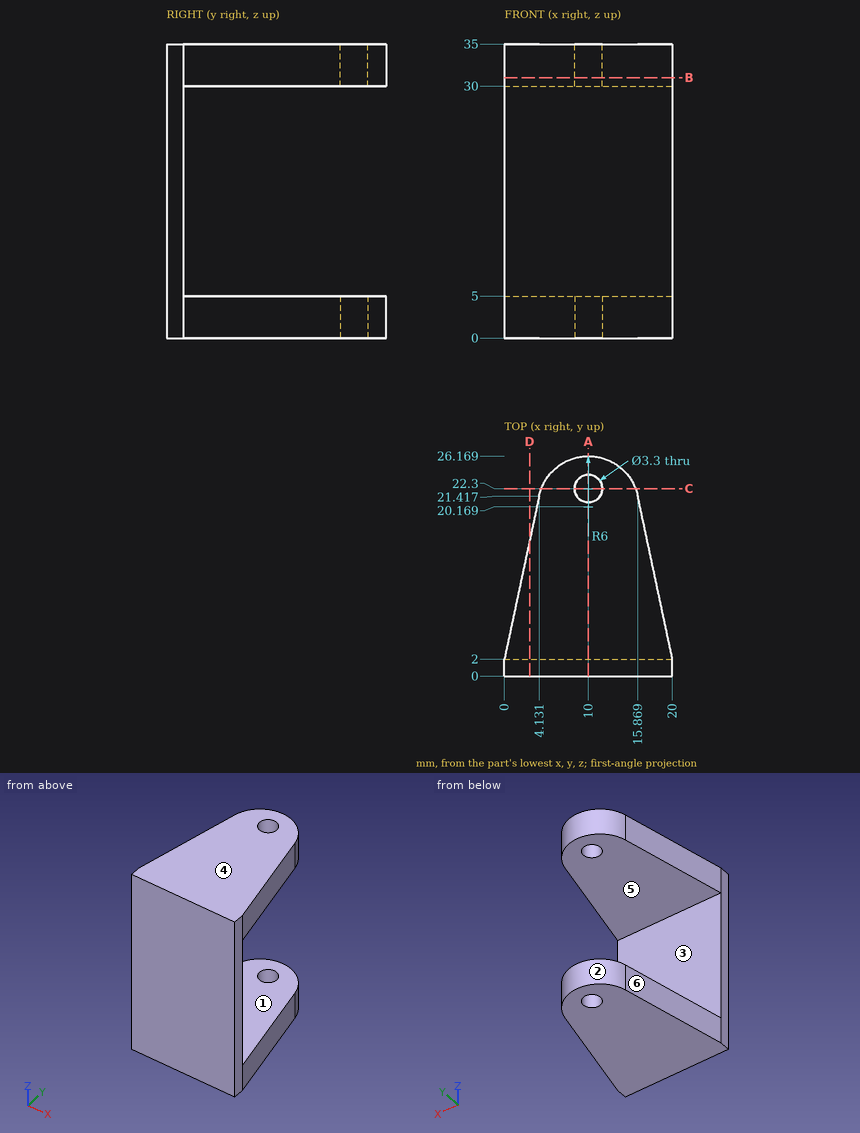
Here's the drawing with two shaded views (mm, measured from the low corner). I have some questions. A direction names the side the tool comes from. Round coordinates to 2 decimals unless told otherwise and drop trailing zeros. Write each loop counter-clockwise with the first axis right and the second up, starting at its lowest first coordinate (ties: lowest second). Pieces come first, ordered by that corner, then holes. Notation, with made-up numbers: M 26,64.25 L 61,64.25 A23 ccw 61,79.25 Z; hole C 15.5,-4 d9. An arc over 180 degrees is marked long. Use CSV: the item, a comma, the result in double quotes.
(1) Imagine slicing it at A-A (x = 10). Write out the boundary of the cut face in (y, z).
Check values:
outline,"M 0,0 L 20.65,0 L 20.65,5 L 2,5 L 2,30 L 20.65,30 L 20.65,35 L 0,35 Z; M 23.95,0 L 26.17,0 L 26.17,5 L 23.95,5 Z; M 23.95,30 L 26.17,30 L 26.17,35 L 23.95,35 Z"
(2) On a 3-axis mill with a long thin cutter (end or side, diameter ignored), from which of +Z, -Z, +X, -X, +Y, -Y can I reach the whole of each face in a straight line? I mean the marked faces 5 and 6. Say none if no direction works.
Check values:
face 5,"+X, -X, +Y"
face 6,"+Z, -Z, -X, +Y"
(3) Imagine slicing it at C-C (y = 22.3). Write out the boundary of the cut face in (x, z).
Check values:
outline,"M 4.39,0 L 8.35,0 L 8.35,5 L 4.39,5 Z; M 4.39,30 L 8.35,30 L 8.35,35 L 4.39,35 Z; M 11.65,0 L 15.61,0 L 15.61,5 L 11.65,5 Z; M 11.65,30 L 15.61,30 L 15.61,35 L 11.65,35 Z"
(4) I need wall thicknesses on line 1 along Z through (x, y) = (9, 14); line 2 along Y through (x, z) = (10, 33.05); line 3 along Y through (x, z) = (13.75, 14.5). Which ranges of each line are inside material? Lowest first, please.
Check values:
line 1,"0 to 5, 30 to 35"
line 2,"0 to 20.65, 23.95 to 26.17"
line 3,"0 to 2"
(5) We'd pull the mould along Z, two halves only. Please class the marked faces 1, 2, 3 and 4: +Z half, -Z half, draft (parallel to the pull), parting line (faces both ways), or undercut.
Check values:
face 1,"undercut"
face 2,"draft"
face 3,"undercut"
face 4,"+Z half"
(6) Imagine slicing it at D-D (x = 3). Write out the boundary of the cut face in (y, z), plus the area to 3 significant figures.
Check values:
outline,"M 0,0 L 16.1,0 L 16.1,5 L 2,5 L 2,30 L 16.1,30 L 16.1,35 L 0,35 Z"
area,"211 mm^2"
(7) Imagine slicing it at B-B (z = 31). Write out the boundary of the cut face in (x, y), plus the area to 3 significant figures.
Check values:
outline,"M 0,0 L 20,0 L 20,2 L 15.87,21.42 A6 ccw 4.13,21.42 L 0,2 Z; hole C 10,22.3 d3.3"
area,"381 mm^2"
(8) I'm going to push flat-ended pins straight in: pin 1 (1.5 mm diameter, centred on y = 4.5, z = 13.5, fed in from +X); pin 2 (1.5 mm diameter, centred on x = 11, z = 20.5, fed in from +Y); pin 3 (8 mm diameter, centred on x = 17, z = 30.5, fed in from +Y) (1 decimal). Where does each tip first touch, or does it pass through?
Check values:
pin 1,"through"
pin 2,"y = 2"
pin 3,"y = 25.4"
